from build123d import *

# Parameters (mm, degrees)
F1_DEPTH  = 25.4
F2_W      = 50.8
F2_H      = 25.4
F3_DEPTH  = 25.4
F5_DEPTH  = 673.1
F4_W      = 1193.8120010341
F4_H      = 25.4
F7_DEPTH  = 25.4
F8_DEPTH  = 279.4
F9_W      = 50.728738308
F9_H      = 76.2
F10_DEPTH = 25.4
F11_W     = 50.8
F11_H     = 76.2
F12_DEPTH = 25.4


# Not quite as in the source:
# - ends of sketch curves that miss each other by under 0.0002 mm in the source are joined


with BuildPart() as f1:
    # F0 (on Top) → F1 (new body)
    with BuildSketch(Plane.XY):
        with BuildLine():
            Line((715.1671976125, 685.8), (-592.9328023875, 685.8))
            ThreePointArc((-592.9328023875, 685.8), (-610.8933146297, 678.3605122421), (-618.3328023875, 660.4))
            Line((-618.3328023875, 660.4), (-618.3328023875, 25.4))
            ThreePointArc((-618.3328023875, 25.4), (-610.8933146297, 7.4394877579), (-592.9328023875, 0))
            Line((-592.9328023875, 0), (715.1671976125, 0))
            ThreePointArc((715.1671976125, 0), (733.1277098546, 7.4394877579), (740.5671976125, 25.4))
            Line((740.5671976125, 25.4), (740.5671976125, 660.4))
            ThreePointArc((740.5671976125, 660.4), (733.1277098546, 678.3605122421), (715.1671976125, 685.8))
        make_face()
    extrude(amount=F1_DEPTH)

    # F2 (on face) → F3 (join)
    with BuildSketch(Plane(origin=(0, 0, 0), x_dir=(1, 0, 0), z_dir=(0, 0, -1))):
        with Locations((-561.1828023875, -114.3)):
            Rectangle(F2_W, F2_H)
        with BuildLine():
            Line((-535.7828023875, -127), (-586.5828023875, -127))
            Line((-586.5828023875, -127), (-586.5828023875, -533.4))
            ThreePointArc((-586.5828023875, -533.4), (-579.1433146297, -551.3605122421), (-561.1828023875, -558.8))
            ThreePointArc((-561.1828023875, -558.8), (-543.2222901454, -551.3605122421), (-535.7828023875, -533.4))
            Line((-535.7828023875, -533.4), (-535.7828023875, -127))
        make_face()
        with BuildLine():
            Line((708.8171976125, -127), (658.0171976125, -127))
            Line((658.0171976125, -127), (658.0171976125, -533.4))
            ThreePointArc((658.0171976125, -533.4), (665.4566853703, -551.3605122421), (683.4171976125, -558.8))
            ThreePointArc((683.4171976125, -558.8), (701.3777098546, -551.3605122421), (708.8171976125, -533.4))
            Line((708.8171976125, -533.4), (708.8171976125, -127))
        make_face()
        with Locations((683.4171976125, -114.3)):
            Rectangle(F2_W, F2_H)
    extrude(amount=F3_DEPTH)

    # F4 (on face) → F5 (join)
    with BuildSketch(Plane(origin=(0, 0, -25.4), x_dir=(1, 0, 0), z_dir=(0, 0, -1))):
        Polygon((-535.7828023875, -127), (-535.7828023875, -101.6), (-586.5828023875, -101.6), (-586.5828023875, -177.8), (-535.7828023875, -177.8), align=None)
        Polygon((708.7579369545, -101.6), (658.0291986465, -101.6), (658.0291986465, -127), (658.0291986465, -177.8), (708.7579369545, -177.8), align=None)
    extrude(amount=F5_DEPTH)

    # F4 (on face) → F7 (join)
    with BuildSketch(Plane(origin=(0, 0, -25.4), x_dir=(1, 0, 0), z_dir=(0, 0, -1))):
        with Locations((61.1231981295, -114.3)):
            Rectangle(F4_W, F4_H)
    extrude(amount=-F7_DEPTH)

    # F4 (on face) → F8 (join)
    with BuildSketch(Plane(origin=(0, 0, -25.4), x_dir=(1, 0, 0), z_dir=(0, 0, -1))):
        with Locations((61.1231981295, -114.3)):
            Rectangle(F4_W, F4_H)
    extrude(amount=F8_DEPTH)

    # F9 (on face) → F10 (join)
    with BuildSketch(Plane(origin=(0, 0, -698.5), x_dir=(1, 0, 0), z_dir=(0, 0, -1))):
        with BuildLine():
            Line((708.7579369545, -177.8), (658.0291986465, -177.8))
            Line((658.0291986465, -177.8), (658.0291986465, -520.7))
            ThreePointArc((658.0291986465, -520.7), (665.4435093373, -538.6352998323), (683.357937235, -546.0999000355))
            Line((683.357937235, -546.0999000355), (683.4291986465, -546.1))
            ThreePointArc((683.4291986465, -546.1), (701.3436262637, -538.6352998323), (708.7579369545, -520.7))
            Line((708.7579369545, -520.7), (708.7579369545, -177.8))
        make_face()
        with Locations((683.3935678005, -139.7)):
            Rectangle(F9_W, F9_H)
        with BuildLine():
            Line((658.0291986465, -50.8), (658.0291986465, -101.6))
            Line((658.0291986465, -101.6), (708.7579369545, -101.6))
            Line((708.7579369545, -101.6), (708.8171976125, -101.6))
            Line((708.8171976125, -101.6), (708.8171976125, -50.8))
            ThreePointArc((708.8171976125, -50.8), (701.3819523594, -32.843731265), (683.4291986452, -25.4000028351))
            Line((683.4291986452, -25.4000028351), (683.4171976125, -25.4))
            ThreePointArc((683.4171976125, -25.4), (665.4644438997, -32.843731265), (658.0291986465, -50.8))
        make_face()
    extrude(amount=F10_DEPTH)

    # F11 (on face) → F12 (join)
    with BuildSketch(Plane(origin=(0, 0, -698.5), x_dir=(1, 0, 0), z_dir=(0, 0, -1))):
        with BuildLine():
            ThreePointArc((-561.1828023875, -25.4), (-579.1433146297, -32.8394877579), (-586.5828023875, -50.8))
            Line((-586.5828023875, -50.8), (-586.5828023875, -101.6))
            Line((-586.5828023875, -101.6), (-535.7828023875, -101.6))
            Line((-535.7828023875, -101.6), (-535.7828023875, -50.8))
            ThreePointArc((-535.7828023875, -50.8), (-543.2222901454, -32.8394877579), (-561.1828023875, -25.4))
        make_face()
        with Locations((-561.1828023875, -139.7)):
            Rectangle(F11_W, F11_H)
        with BuildLine():
            Line((-535.7828023875, -177.8), (-586.5828023875, -177.8))
            Line((-586.5828023875, -177.8), (-586.5828023875, -520.7))
            ThreePointArc((-586.5828023875, -520.7), (-579.1433146297, -538.6605122421), (-561.1828023875, -546.1))
            ThreePointArc((-561.1828023875, -546.1), (-543.2222901454, -538.6605122421), (-535.7828023875, -520.7))
            Line((-535.7828023875, -520.7), (-535.7828023875, -177.8))
        make_face()
    extrude(amount=F12_DEPTH)


solid = f1.part
Read the model definition and answer for the solid it produces. Units are mm, in the model's axes. A direction names the side the tool comes from. Round coordinates to 2 decimals unless told otherwise and drop trailing zeros. Loops run counter-clockwise (first coordinate to the right, second up) from the corner with the lowest first, then second, coordinate; pieces in that order, holes last.
Q1. Section B-B on y = 467 is taken. Write down the section's boundary in (x, z), and give its area (3 significant figures).
Q2. Section C-C on x = -223 is taken. Write down the section's boundary in (y, z), and give its area (3 significant figures).
Q3. Consider probe 1 along X at (y, z) = (105.5, -456); probe 2 along Z at (x, y) = (-68.5, 237); probe 3 along Y at (x, z) = (-102.5, -70.5). Determine where each line is inside the solid, lowest interval first.
Q4. Section A-A on z = -345 is taken. Write down the section's boundary in (x, y).
Q5. Determine the mould class of faces 1 (the face through (708.758, 172, -425)), 2 (the face through (683, 378, -25.4)), 3 (the face through (52, 348, 0)) for opening direction X: released by +X, released by -X, zero draft, split by the parting line, or undercut.
Q6. Section D-D on z = -248 is taken. Write down the section's boundary in (x, y), and give its area (3 significant figures).
Q7. Which of the six approach directions +Z, -Z, +X, -X, +Y, -Y give full straight-line access (tool end or side, diameter ignored) to faces 4 (the face through (-562, 366, -25.4)), 5 (the face through (-586.583, 166, -360)), 6 (the face through (683, 63, -698.5)), 7 (the face through (-562, 282, -723.9)), 8 (the face through (53, 127, -150))?
Q8. Each of these flat-tipped pins is pushed along its axis until it touches: pin 1 (10 mm diameter, centred on x = -60.5, y = 556.5, fed in from -Z); pin 2 (7.5 mm diameter, centred on x = -96.5, y = 113.5, fed in from -Z); pin 3 (20.5 mm diameter, centred on y = 403.5, z = -10.5, fed in from -X). Where does it stop, or does it pass through?
Output:
1. outline: (-618.33, 0) - (-586.58, 0) - (-586.58, -25.4) - (-535.78, -25.4) - (-535.78, 0) - (658.02, 0) - (658.02, -25.4) - (708.82, -25.4) - (708.82, 0) - (740.57, 0) - (740.57, 25.4) - (-618.33, 25.4) - close; (-586.58, -723.9) - (-535.78, -723.9) - (-535.78, -698.5) - (-586.58, -698.5) - close; (658.03, -723.9) - (708.76, -723.9) - (708.76, -698.5) - (658.03, -698.5) - close
1. area: 39,700 mm2
2. outline: (0, 0) - (101.6, 0) - (101.6, -304.8) - (127, -304.8) - (127, 0) - (685.8, 0) - (685.8, 25.4) - (0, 25.4) - close
2. area: 25,200 mm2
3. probe 1: x = -586.58 to -535.78, 658.03 to 708.76
3. probe 2: z = 0 to 25.4
3. probe 3: y = 101.6 to 127
4. outline: (-586.58, 101.6) - (-535.78, 101.6) - (-535.78, 177.8) - (-586.58, 177.8) - close; (658.03, 101.6) - (708.76, 101.6) - (708.76, 177.8) - (658.03, 177.8) - close
5. face 1: released by +X
5. face 2: zero draft
5. face 3: undercut
6. outline: (-586.58, 101.6) - (708.76, 101.6) - (708.76, 177.8) - (658.03, 177.8) - (658.03, 127) - (-535.78, 127) - (-535.78, 177.8) - (-586.58, 177.8) - close
6. area: 38,100 mm2
7. face 4: +X, -X, +Y
7. face 5: -Z, -X, +Y, -Y
7. face 6: +X, -X, -Y
7. face 7: -Z, +X, -X, +Y, -Y
7. face 8: -Z, +Y
8. pin 1: stops at z = 0
8. pin 2: stops at z = -304.8
8. pin 3: stops at x = -586.58
